Source: CAD feature listing. Evaluate the final solid. Frame: model axes, mm. Coordinates: 2 decimals unless noted, no trailing zeros. Order: outer loops, then holes, each group sorted by start corner. A loop starts at its lowest first (then second) coordinate and runs counter-clockwise, first axis right, second up.
Autodesk Inventor part; units mm, degrees
ref_plane "Work Plane2" through (0, 0, 235.7438) normal (0, 0, 1) x (1, 0, 0)
ref_plane "YZ Plane" through (0, 0, 0) normal (1, 0, 0) x (0, 1, 0)
ref_plane "XZ Plane" through (0, 0, 0) normal (0, 1, 0) x (-1, 0, 0)
sketch "Sketch1" plane through (0, 0, 0) normal (0, 0, 1) x (1, 0, 0)
  circle A0 centre (0, 0) radius 406.4
  circle A1 centre (0, 0) radius 387.35
  dimension "d0" = 812.8
  dimension "d1" = 774.7
extrude "Extrusion1" add sketch "Sketch1" along normal blind 267.4937
chamfer "Chamfer1" distance 17.4625 angle 37.5 1 edges at (-406.4, 0, 0) measured on face at (-399.72, -9.4497, 0)
ref_plane "Work Plane2" through (0, 0, 235.7438) normal (0, 0, 1) x (1, 0, 0)
ref_plane "Work Plane1" through (0, 0, 216.6938) normal (0, 0, 1) x (1, 0, 0)
split_face "Split1"
split_face "Split2"
chamfer "Chamfer2" distance 0.7937 angle 45 1 edges at (-387.35, 0, 267.4937)
properties part number "A1-19037-100-03 32in pipe" material "Steel, Mild"
1. Ray query, line 1 (Y direction, x = 0, z = 194); line 2 (X direction, y = -2, z = 221); line 3 (Y direction, x = -8.5, z = 126.5). Return the intervals inside material, ascending.
Findings:
line 1: y = -406.4 to -387.35, 387.35 to 406.4
line 2: x = -406.4 to -387.34, 387.34 to 406.4
line 3: y = -406.31 to -387.26, 387.26 to 406.31
2. Section query C-C on z = 164. Return loops of the section in (x, y).
Findings:
outline: circle Ø812.8 at (0, 0); hole circle Ø774.7 at (0, 0)
3. Draft query along Y for faces 1 (the face through (-88.1, 396.736, 138.668)), 2 (the face through (-83.97, 378.14, 131.48)), 3 (the face through (359, -149, 267.494)). Return one class per face: released by +Y, released by -Y, zero draft, split by the parting line, or undercut.
Findings:
face 1: split by the parting line
face 2: undercut
face 3: zero draft
4. Section query A-A on y = 0. Return loops of the section in (x, z).
Findings:
outline: (-406.4, 13.4) - (-388.94, 0) - (-387.35, 0) - (-387.35, 266.7) - (-388.14, 267.49) - (-406.4, 267.49) - close; (387.35, 0) - (388.94, 0) - (406.4, 13.4) - (406.4, 267.49) - (388.14, 267.49) - (387.35, 266.7) - close
5. Pin query (flat end, axial travel): P1, Ø10, axis at x = -257.5, z = 235, coming from the +Y side; P2, Ø4, axis at y = 152.5, z = 216.5, coming from the -X side; P3, Ø8, axis at y = -27.5, z = 236.5, coming from the -X side. Return the tip coordinate at first contact, or that it passes through.
Findings:
P1: stops at y = 318.44
P2: stops at x = -377.51
P3: stops at x = -405.72
